Read the model definition and answer for the solid it produces. Units are mm, in the model's axes. Coordinates: 2 decimals unless noted, no trailing zeros. Loops run counter-clockwise (first coordinate to the right, second up) from the corner with the lowest first, then second, coordinate; pieces in that order, holes last.
from build123d import *

# Parameters (mm, degrees)
SKETCH2_R           = 1.75
SKETCH2_R_2         = 9
SKETCH2_R_3         = 20
SKETCH2_R_4         = 10
SKETCH2_R_5         = 6
BOSS_EXTRUDE1_DEPTH = 2.5
FILLET1_R           = 1


with BuildPart() as part:
    # Sketch2 → Boss-Extrude1 (new, symmetric)
    # profile 1 of 6: a face of its own
    with BuildSketch(Plane.XY):
        with BuildLine():
            ThreePointArc((4.931171461, 183.44633077), (-12.782697282, 203.949164453), (6.192423965, 223.290625322))
            ThreePointArc((6.192423965, 223.290625322), (-74.438391307, 216.57190759), (-154.465632764, 204.650910815))
            ThreePointArc((-154.465632764, 204.650910815), (-147.086827714, 202.707602973), (-143.852204973, 195.796711203))
            ThreePointArc((-143.852204973, 195.796711203), (-146.265984708, 189.663057919), (-152.212583331, 186.819468634))
            ThreePointArc((-152.212583331, 186.819468634), (-73.562569521, 188.773026517), (4.931171461, 183.44633077))
        make_face()
        with Locations((-127.852204973, 199.130573991)):
            Circle(SKETCH2_R, mode=Mode.SUBTRACT)
        with Locations((-24.542709853, 204.413331435)):
            Circle(SKETCH2_R, mode=Mode.SUBTRACT)
    # profile 2 of 6: a face of its own
    with BuildSketch(Plane.XY):
        with Locations((-152.852204973, 195.796711203)):
            Circle(SKETCH2_R_2)
        with Locations((-152.852204973, 195.796711203)):
            Circle(SKETCH2_R, mode=Mode.SUBTRACT)
    # profile 3 of 6: a face of its own
    with BuildSketch(Plane.XY):
        with Locations((7.207290147, 203.316390753)):
            Circle(SKETCH2_R_3)
        with Locations((7.207290147, 203.316390753)):
            Circle(SKETCH2_R_4, mode=Mode.SUBTRACT)
    # profile 4 of 6: a face of its own
    with BuildSketch(Plane.XY):
        with Locations((7.207290147, 203.316390753)):
            Circle(SKETCH2_R_4)
        with Locations((7.207290147, 203.316390753)):
            Circle(SKETCH2_R, mode=Mode.SUBTRACT)
    # profile 5 of 6: a face of its own
    with BuildSketch(Plane.XY):
        with Locations((61.147795027, 205.850544138)):
            Circle(SKETCH2_R_5)
        with Locations((61.147795027, 205.850544138)):
            Circle(SKETCH2_R, mode=Mode.SUBTRACT)
    # profile 6 of 6: a face of its own
    with BuildSketch(Plane.XY):
        with BuildLine():
            ThreePointArc((14.489310329, 221.943580076), (23.724559953, 214.593792855), (27.207290147, 203.316390753))
            ThreePointArc((27.207290147, 203.316390753), (24.972572156, 194.129728945), (18.767814631, 186.99602698))
            ThreePointArc((18.767814631, 186.99602698), (38.842152118, 196.840042673), (60.99636255, 199.852455425))
            ThreePointArc((60.99636255, 199.852455425), (55.152157086, 206.079292207), (61.453820667, 211.842734748))
            ThreePointArc((61.453820667, 211.842734748), (37.564582261, 215.000863469), (14.489310329, 221.943580076))
        make_face()
    extrude(amount=BOSS_EXTRUDE1_DEPTH, both=True)

    # Fillet1
    fillet1_edges = [part.edges().sort_by_distance(p)[0] for p in [
        (10.412432506, 223.057896837, -2.5),
        (37.564582261, 215.000863469, -2.5),
        (67.143432968, 205.621796069, -2.5),
        (38.842152118, 196.840042673, -2.5),
        (12.177213039, 183.94373305, -2.5),
        (-73.562569521, 188.773026517, -2.5),
        (-161.781211479, 194.66850784, -2.5),
        (-74.438391307, 216.57190759, 2.5),
        (-74.438391307, 216.57190759, -2.5),
        (-161.781211479, 194.66850784, 2.5),
        (-73.562569521, 188.773026517, 2.5),
        (12.177213039, 183.94373305, 2.5),
        (38.842152118, 196.840042673, 2.5),
        (67.143432968, 205.621796069, 2.5),
        (37.564582261, 215.000863469, 2.5),
        (10.412432506, 223.057896837, 2.5),
    ]]
    fillet(fillet1_edges, radius=FILLET1_R)


solid = part.part
Item 1: Find the intervals of material crossed by line 1 along X through (y, z) = (203.5, 1.2); line 2 along Z through (x, y) = (55, 200.5); line 3 along Y through (x, z) = (-128, 0.65), in increasing order.
Numbers:
line 1: x = -157.51 to -26.04, -23.05 to 5.47, 8.95 to 66.67
line 2: z = -2.47 to 2.47
line 3: y = 188.2 to 197.39, 200.87 to 209.18
Item 2: Determine the mould class of faces 1 (the face through (-154.24, 194.73, -0.04)), 2 (the face through (-49, 204, -2.5)), 3 (the face through (12.08, 183.92, 0.02)) for opening direction Y: released by +Y, released by -Y, zero draft, split by the parting line, or undercut.
Numbers:
face 1: undercut
face 2: zero draft
face 3: released by -Y
Item 3: Given pin 1 (1 mm diameter, centred on x = -27.5, z = 0, fed in from +Y); pin 2 (3 mm diameter, centred on x = 61.15, y = 205.85, fed in from +Z); pin 3 (1.5 mm diameter, centred on x = -101, z = -1, fed in from -Y), each flat-ended and moving along its own axis, determine where each tip first touches the part or whether it passes through.
Numbers:
pin 1: stops at y = 221.16
pin 2: passes through
pin 3: stops at y = 188.91
Item 4: A cutting plane is placed at A-A on z = -0.7. Determine the outline of the cut face in (x, y), then the cut area to 3 significant figures.
Numbers:
outline: (-154.47, 204.65) arc R9 ccw to (-152.21, 186.82) arc R850 cw to (4.93, 183.45) arc R20 ccw to (18.77, 187) arc R70 cw to (61, 199.85) arc R6 ccw to (61.45, 211.84) arc R150 cw to (14.49, 221.94) arc R20 ccw to (6.19, 223.29) arc R1250 ccw to start; hole circle Ø3.5 at (-152.85, 195.8); hole circle Ø3.5 at (-127.85, 199.13); hole circle Ø3.5 at (-24.54, 204.41); hole circle Ø3.5 at (7.21, 203.32); hole circle Ø3.5 at (61.15, 205.85)
area: 5,930 mm2
